Input: part model. Units: mm. Frame: model coordinates. A direction names the side the tool comes from. Give positions to 0.01 mm unless a question says otherwise; leave off trailing zeros. Order: outer loops, then holes, each group sorted by start corner. A loop starts at its lowest first (then second) coordinate and runs counter-clockwise, first axis right, second up. Notation, with made-up numbers: (-36.75, 68.25) - (-4.75, 68.25) arc R17 ccw to (-4.75, 80.25) - close; hole circle Ø2 at (11.25, 13). An arc over 180 degrees is marked (long way). Use a Markdown table: item, result.
from build123d import *

# Parameters (mm, degrees)
SKETCH1_W           = 20
SKETCH1_H           = 10
BOSS_EXTRUDE1_DEPTH = 2
SKETCH4_R           = 3
BOSS_EXTRUDE2_DEPTH = 4


with BuildPart() as part:
    # Sketch1 → Boss-Extrude1 (new body)
    with BuildSketch(Plane(origin=(0, 0, 0), x_dir=(1, 0, 0), z_dir=(0, 1, 0))):
        with Locations((0, -5)):
            Rectangle(SKETCH1_W, SKETCH1_H)
    extrude(amount=BOSS_EXTRUDE1_DEPTH)

    # Sketch4 → Boss-Extrude2 (add)
    with BuildSketch(Plane(origin=(6, 0, 0), x_dir=(0, 0, -1), z_dir=(1, 0, 0))):
        with BuildLine():
            Line((0, 2), (1.5, 4.814384898))
            ThreePointArc((1.5, 4.814384898), (9.181980515, 7.996365414), (6, 0.314384898))
            Line((6, 0.314384898), (0, -0.014042226))
            Line((0, -0.014042226), (0, 2))
        make_face()
        with Locations((6, 4.814384898)):
            Circle(SKETCH4_R, mode=Mode.SUBTRACT)
    boss_extrude2 = extrude(amount=BOSS_EXTRUDE2_DEPTH)

    # Mirror1: Boss-Extrude2 across plane
    add(boss_extrude2.mirror(Plane(origin=(0, 0, 0), x_dir=(0, 0, 1), z_dir=(1, 0, 0))))


solid = part.part
1. Set-up query: faces 1 (the face through (-10, 3.7, -2.7)), 2 (the face through (6, 3.7, -3)), 3 (the face through (0, 2, 5)). Return all of +Z, -Z, +X, -X, +Y, -Y with unobstructed straight access to the full face (end or side cutting, diameter ignored); none if empty.
Response:
| item | result |
|---|---|
| face 1 | +Z, -Z, -X, +Y, -Y |
| face 2 | -Z, +Y, -Y |
| face 3 | +Z, +X, -X, +Y |
2. Section query D-D (y = 1). Return loops of the section in (x, z).
Response:
| item | result |
|---|---|
| outline | (-10, -8.39) - (-6, -8.39) - (-6, 0) - (6, 0) - (6, -8.39) - (10, -8.39) - (10, 10) - (-10, 10) - close |
3. Material intervals for line 1 along X through (y, z) = (8, -5.25); line 2 along Y through (x, z) = (-8.95, -6); line 3 along Y through (x, z) = (-4.5, 1.5), sorted ascending.
Response:
| item | result |
|---|---|
| line 1 | x = -10 to -6, 6 to 10 |
| line 2 | y = 0.31 to 1.81, 7.81 to 9.31 |
| line 3 | y = 0 to 2 |
4. Section query B-B (y = 5.75). Return loops of the section in (x, z), then the cut area to 3 significant figures.
Response:
| item | result |
|---|---|
| outline | (-10, -10.4) - (-6, -10.4) - (-6, -8.85) - (-10, -8.85) - close; (-10, -3.15) - (-6, -3.15) - (-6, -1.6) - (-10, -1.6) - close; (6, -10.4) - (10, -10.4) - (10, -8.85) - (6, -8.85) - close; (6, -3.15) - (10, -3.15) - (10, -1.6) - (6, -1.6) - close |
| area | 24.8 mm^2 |
5. Pin query (flat end, axial travel): pin 1 (4 mm diameter, centred on x = -0.5, y = 5, fed in from +Z); pin 2 (4 mm diameter, centred on x = -5, z = 4.5, fed in from +Y); pin 3 (5 mm diameter, centred on x = 7, z = -5.5, fed in from -Y); pin 4 (1 mm diameter, centred on x = 6.5, y = 4, fed in from +Z). Return the tip coordinate at first contact, or that it passes through.
Response:
| item | result |
|---|---|
| pin 1 | passes through |
| pin 2 | stops at y = 2 |
| pin 3 | stops at y = 0.15 |
| pin 4 | stops at z = -0.8 |
6. Section query C-C (z = -8.5). Return loops of the section in (x, y).
Response:
| item | result |
|---|---|
| outline | (-10, 1.07) - (-6, 1.07) - (-6, 3.16) - (-10, 3.16) - close; (-10, 6.47) - (-6, 6.47) - (-6, 8.56) - (-10, 8.56) - close; (6, 1.07) - (10, 1.07) - (10, 3.16) - (6, 3.16) - close; (6, 6.47) - (10, 6.47) - (10, 8.56) - (6, 8.56) - close |
7. Mould query, pull axis Z, two halves, no side actions, for faces 4 (the face through (7.972, 1.886, -5.35)), 5 (the face through (7.972, 8.1, -9.075)), 6 (the face through (10, 3.7, -2.7)), 7 (the face through (-7.972, 1.886, -5.35)). Classes: pulls with the +Z half, pulls with the -Z half, needs draft (parallel to the pull), parting line crosses it, or undercut.
Response:
| item | result |
|---|---|
| face 4 | undercut |
| face 5 | parting line crosses it |
| face 6 | needs draft |
| face 7 | undercut |
